from build123d import *

# Parameters (mm, degrees)
SKIZZE1_R                       = 1
SKIZZE1_R_2                     = 2
AUFSATZ_LINEAR_AUSTRAGEN1_DEPTH = 3
SKIZZE2_R                       = 2
SCHNITT_LINEAR_AUSTRAGEN1_DEPTH = 45.821869662
VERRUNDUNG1_R                   = 5


with BuildPart() as part:
    # Skizze1 → Aufsatz-Linear austragen1 (new body)
    with BuildSketch(Plane.XY):
        with BuildLine():
            Line((40, 20), (0, 20))
            ThreePointArc((0, 20), (-20, 0), (0, -20))
            Line((0, -20), (40, -20))
            Line((40, -20), (40, 20))
        make_face()
        Circle(SKIZZE1_R, mode=Mode.SUBTRACT)
        with Locations((35, 15)):
            Circle(SKIZZE1_R_2, mode=Mode.SUBTRACT)
        with Locations((35, -15)):
            Circle(SKIZZE1_R_2, mode=Mode.SUBTRACT)
    extrude(amount=AUFSATZ_LINEAR_AUSTRAGEN1_DEPTH)

    # Skizze2 → Schnitt-Linear austragen1 (cut, through all)
    with BuildSketch(Plane(origin=(0, 0, 0), x_dir=(-1, 0, 0), z_dir=(0, 0, -1))):
        with Locations((-10.8, 0)):
            Circle(SKIZZE2_R)
        with Locations((5.4, 9.353074361)):
            Circle(SKIZZE2_R)
        with Locations((5.4, -9.353074361)):
            Circle(SKIZZE2_R)
    extrude(amount=-SCHNITT_LINEAR_AUSTRAGEN1_DEPTH, mode=Mode.SUBTRACT)

    # Verrundung1
    verrundung1_edges = [part.edges().sort_by_distance(p)[0] for p in [
        (40, 20, 1.5),
        (40, -20, 1.5),
    ]]
    fillet(verrundung1_edges, radius=VERRUNDUNG1_R)


solid = part.part
Here's how the part is built. I have some questions about the finished solid (model axes, mm). Round coordinates to 2 decimals unless told otherwise and drop trailing zeros. Write each loop counter-clockwise with the first axis right and the second up, starting at its lowest first coordinate (ties: lowest second). Pieces come first, ordered by that corner, then holes. Notation, with made-up numbers: (74.25, 26) -> (120.25, 26) arc R17 ccw to (120.25, 48) -> close; hole circle Ø10 at (25, 3). An arc over 180 degrees is marked (long way). One line per item, written item: value.
1) I'm going to push a flat-ended pin straight in: pin 1 Ø2.5 at (x, y) = (10.8, 0) entering from -Z. Where does the tip first touch, or does it pass through?
Filled sheet:
pin 1: passes through
2) Suppose I cut it at C-C on y = 12. List the corners of the cut face in (x, z) for me, plus the area to 3 significant figures.
Filled sheet:
outline: (-16, 0) -> (40, 0) -> (40, 3) -> (-16, 3) -> close
area: 168 mm2
3) Suppose I cut it at B-B on z = 0.85. List the corners of the cut face in (x, y) for me.
Filled sheet:
outline: (0, -20) -> (35, -20) arc R5 ccw to (40, -15) -> (40, 15) arc R5 ccw to (35, 20) -> (0, 20) arc R20 ccw to start; hole circle Ø4 at (-5.4, -9.35); hole circle Ø4 at (-5.4, 9.35); hole circle Ø2 at (0, 0); hole circle Ø4 at (10.8, 0); hole circle Ø4 at (35, -15); hole circle Ø4 at (35, 15)
4) If I drill on line 1 (Y direction, x = 35, z = 1.4); line 2 (X direction, y = -0.5, z = 1.6); line 3 (Y direction, x = -5.4, z = 0.6), over which ranges is the centre line in solid material (lowest first)? Write a range as [from, to].
Filled sheet:
line 1: y = [-20, -17], [-13, 13], [17, 20]
line 2: x = [-19.99, -0.87], [0.87, 8.86], [12.74, 40]
line 3: y = [-19.26, -11.35], [-7.35, 7.35], [11.35, 19.26]
5) We'd pull the mould along X, two halves only. Please class faces 1 (the face through (-20, 0, 1)), 2 (the face through (18, 20, 1)), 3 (the face through (-3.813, -10.57, 1.479)), 4 (the face through (38, 19, 2)): released by +X, released by -X, zero draft, split by the parting line, or undercut.
Filled sheet:
face 1: released by -X
face 2: zero draft
face 3: undercut
face 4: released by +X
6) Suppose I cut it at A-A on y = 0. List the corners of the cut face in (x, z) for me.
Filled sheet:
outline: (-20, 0) -> (-1, 0) -> (-1, 3) -> (-20, 3) -> close; (1, 0) -> (8.8, 0) -> (8.8, 3) -> (1, 3) -> close; (12.8, 0) -> (40, 0) -> (40, 3) -> (12.8, 3) -> close
